Can you work these out from the model? Positions are in its coordinate system, mm. A direction names the side the tool comes from. Coordinates: 2 decimals unless noted, no trailing zeros. Order: outer loops, then holes, each group sorted by start corner. A loop starts at its lowest first (then second) coordinate and runs counter-clockwise, first axis right, second up. Notation, with made-up numbers: (81, 48.25) - (87, 48.25) arc R15 cw to (87, 77.25) - close; hole circle Ø4 at (-39.75, 79.25). An arc over 180 degrees is marked (long way). Use a Markdown table: item, result. Add a question column.
(1) I want a section at A-A (x = -5.5). List the corners of the cut face in (y, z) for me.
(2) For pin 1 Ø2 at (y, z) = (-4.5, -35.5) entering from -X; pin 2 Ø4 at (y, z) = (-4.5, 3.5) entering from -X; pin 3 Ø5 at (x, z) = (32.5, -8.5) entering from -Y, each with a flat end and sliding along its axis, tell me the tip position at first contact or that it passes through.
(3) I want a section at D-D (y = -2.25). List the corners of the cut face in (x, z) for me.
(4) We'd pull the mould along X, two halves only. Please class faces 4 (the flat face through (27, 0, 8)), 5 (the cylindrical face through (-39.05, -3.5, -8.67)), 6 (the flat face through (-29.943, -4.6, -17.263)): pulls with the +X half, pulls with the -X half, needs draft (parallel to the pull), parting line crosses it, or undercut.
(5) I want a section at C-C (x = -16.5). List the corners of the cut face in (y, z) for me.
(6) I want a section at B-B (z = 8.5). List the corners of the cut face in (x, y) for me.
(7) On a 3-axis mill with a long thin cutter (end or side, diameter ignored), from which of +Z, -Z, +X, -X, +Y, -Y can I reach the whole of each face in a straight line? I mean faces 1 (the cylindrical face through (-14.814, -0.493, -27.504)), 2 (the flat face through (-40, -7.1, 4)), 3 (the flat face through (-29.92, -4.6, 17.3)). Say none if no direction works.
(8) If I drill on L1, parallel to X at y = -0.65, z = 0; L2, parallel to Y at x = -28, z = -12; L3, parallel to X at y = -7.5, z = -4.5, over which ranges is the centre line in solid material (lowest first)? Write a range as [from, to].
```python
from build123d import *

# Parameters (mm, degrees)
SKETCH_1_R               = 40
SKETCH_1_R_2             = 28
SKETCH_1_R_3             = 2
EXTRUDE_1_DEPTH          = 1
SKETCH_1_3_R             = 40
SKETCH_1_3_R_2           = 39
EXTRUDE_2_DEPTH          = 7.1
SKETCH_2_R               = 49.5
SKETCH_2_R_2             = 39
EXTRUDE_3_DEPTH          = 1
RIB_1_REACH              = 72.471
SKETCH_4_WALL_W          = 154.404684446
SKETCH_4_WALL_H          = 3
PATTERN_CIRCULAR_1_COUNT = 6


with BuildPart() as part:
    # Sketch 1 → Extrude 1 (new body)
    with BuildSketch(Plane(origin=(0, 0, 0), x_dir=(1, 0, 0), z_dir=(0, 1, 0))):
        with Locations(Location((0, 0, 0), (0, 0, 270))):
            Circle(SKETCH_1_R)
        with Locations(Location((0, 0, 0), (0, 0, 270))):
            Circle(SKETCH_1_R_2, mode=Mode.SUBTRACT)
        with Locations(Location((33, 0, 0), (0, 0, 270))):
            Circle(SKETCH_1_R_3, mode=Mode.SUBTRACT)
        with Locations(Location((16.5, -28.578838325, 0), (0, 0, 270))):
            Circle(SKETCH_1_R_3, mode=Mode.SUBTRACT)
        with Locations(Location((-16.5, -28.578838325, 0), (0, 0, 270))):
            Circle(SKETCH_1_R_3, mode=Mode.SUBTRACT)
        with Locations(Location((-33, 0, 0), (0, 0, 270))):
            Circle(SKETCH_1_R_3, mode=Mode.SUBTRACT)
        with Locations(Location((-16.5, 28.578838325, 0), (0, 0, 270))):
            Circle(SKETCH_1_R_3, mode=Mode.SUBTRACT)
        with Locations(Location((16.5, 28.578838325, 0), (0, 0, 270))):
            Circle(SKETCH_1_R_3, mode=Mode.SUBTRACT)
    extrude(amount=-EXTRUDE_1_DEPTH)

    # Sketch 1_3 → Extrude 2 (add)
    with BuildSketch(Plane(origin=(0, 0, 0), x_dir=(1, 0, 0), z_dir=(0, 1, 0))):
        with Locations(Location((0, 0, 0), (0, 0, 270))):
            Circle(SKETCH_1_3_R)
        with Locations(Location((0, 0, 0), (0, 0, 270))):
            Circle(SKETCH_1_3_R_2, mode=Mode.SUBTRACT)
    extrude(amount=-EXTRUDE_2_DEPTH)

    # Sketch 2 → Extrude 3 (add)
    with BuildSketch(Plane.XZ.offset(7.1)):
        with Locations(Location((0, 0, 0), (0, 0, 270))):
            Circle(SKETCH_2_R)
        with Locations(Location((0, 0, 0), (0, 0, 90))):
            Circle(SKETCH_2_R_2, mode=Mode.SUBTRACT)
    extrude(amount=EXTRUDE_3_DEPTH)

    # Sketch 4 wall → Rib 1 (add, up to next)
    with BuildSketch(Plane(origin=(0, -4.55, -34.5), x_dir=(0, 0.619361407728, 0.785106009796), z_dir=(0, -0.785106009796, 0.619361407728)), mode=Mode.PRIVATE) as rib_1_sk1:
        Rectangle(SKETCH_4_WALL_W, SKETCH_4_WALL_H)
    rib_1_tool1 = extrude(rib_1_sk1.sketch, amount=-RIB_1_REACH, mode=Mode.PRIVATE) - part.part
    rib_1 = rib_1_tool1.solids().sort_by_distance((0, -4.55, -34.5))[0]
    add(rib_1)

    # Pattern Circular 1: Rib 1 ×6 about axis
    pattern_circular_1_axis = Axis((0, 0, 0), (0, 1, 0))
    for i in range(1, PATTERN_CIRCULAR_1_COUNT):
        add(rib_1.rotate(pattern_circular_1_axis, i * 360 / PATTERN_CIRCULAR_1_COUNT))


solid = part.part
```
Answers follow:
| question | item | result |
|---|---|---|
| 1 | outline | (-8.1, -49.19) - (-7.1, -49.19) - (-7.1, -39.62) - (0, -39.62) - (0, -27.45) - (-1, -27.45) - (-1, -38.61) - (-8.1, -38.61) - close; (-8.1, 38.61) - (-1, 38.61) - (-1, 27.45) - (0, 27.45) - (0, 39.62) - (-7.1, 39.62) - (-7.1, 49.19) - (-8.1, 49.19) - close |
| 2 | pin 1 | stops at x = -20.24 |
| 2 | pin 2 | stops at x = -39.97 |
| 2 | pin 3 | stops at y = -1 |
| 3 | outline | circle Ø80 at (0, 0); hole (-34.5, -18.19) - (-28.1, -14.49) - (-26.6, -17.09) - (-33, -20.78) arc R39 ccw to (-1.5, -38.97) - (-1.5, -31.58) - (1.5, -31.58) - (1.5, -38.97) arc R39 ccw to (33, -20.78) - (26.6, -17.09) - (28.1, -14.49) - (34.5, -18.19) arc R39 ccw to (34.5, 18.19) - (28.1, 14.49) - (26.6, 17.09) - (33, 20.78) arc R39 ccw to (1.5, 38.97) - (1.5, 31.58) - (-1.5, 31.58) - (-1.5, 38.97) arc R39 ccw to (-33, 20.78) - (-26.6, 17.09) - (-28.1, 14.49) - (-34.5, 18.19) arc R39 ccw to start |
| 4 | face 4 | needs draft |
| 4 | face 5 | parting line crosses it |
| 4 | face 6 | undercut |
| 5 | outline | (-8.1, -46.67) - (-7.1, -46.67) - (-7.1, -36.44) - (0, -36.44) - (0, -30.58) - (-1, -30.58) - (-1, -35.34) - (-8.1, -35.34) - close; (-8.1, 35.34) - (-1, 35.34) - (-1, 30.58) - (0, 30.58) - (0, 36.44) - (-7.1, 36.44) - (-7.1, 46.67) - (-8.1, 46.67) - close; (-1, -26.58) - (0, -26.58) - (0, -22.62) - (-1, -22.62) - close; (-1, 22.62) - (0, 22.62) - (0, 26.58) - (-1, 26.58) - close |
| 6 | outline | (-48.76, -8.1) - (-38.06, -8.1) - (-38.06, -1) - (-26.68, -1) - (-26.68, 0) - (-39.09, 0) - (-39.09, -7.1) - (-48.76, -7.1) - close; (26.68, -1) - (38.06, -1) - (38.06, -8.1) - (48.76, -8.1) - (48.76, -7.1) - (39.09, -7.1) - (39.09, 0) - (26.68, 0) - close |
| 7 | face 1 | +Y, -Y |
| 7 | face 2 | +Y |
| 7 | face 3 | -Y |
| 8 | L1 | x = [-40, -35], [-31, -28], [28, 31], [35, 40] |
| 8 | L2 | y = [-1, 0] |
| 8 | L3 | x = [-49.3, -38.74], [38.74, 49.3] |
